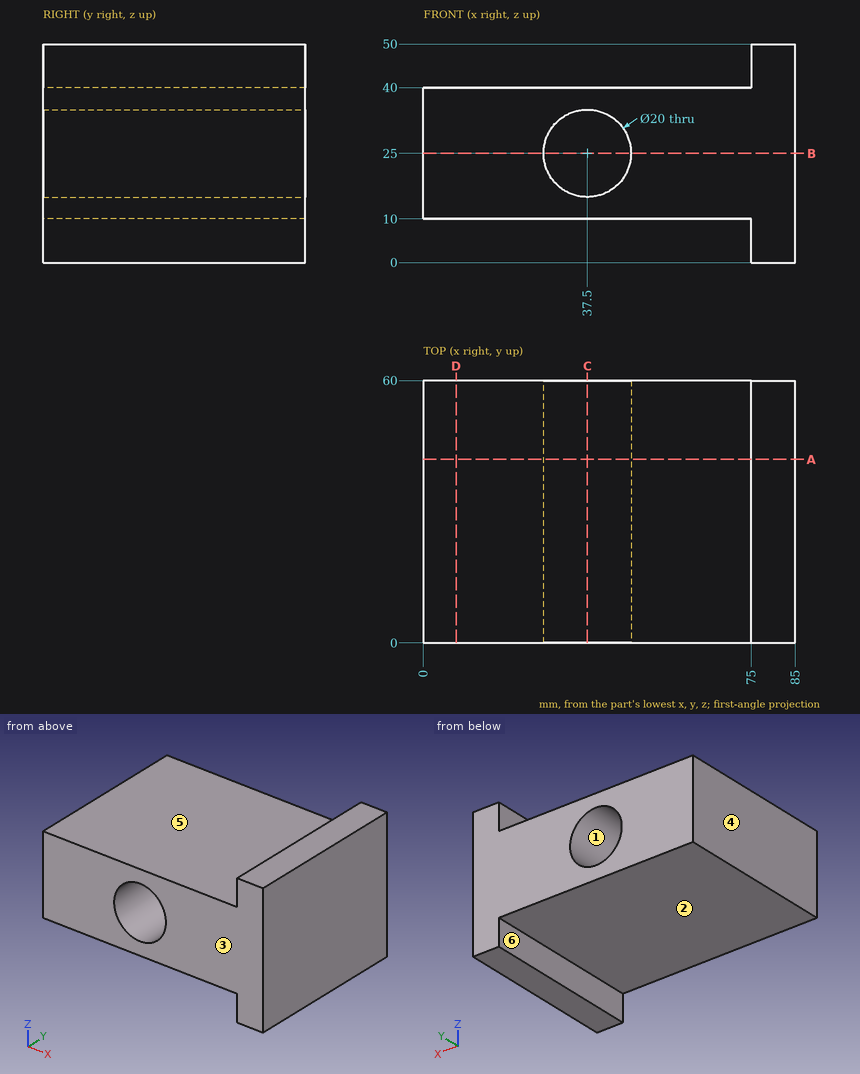
The figure shows three views and two pictorial views of one solid part (mm, origin at its lowest corner). Answer the questions. A direction names the side the tool comes from. Coordinates: 2 decimals unless noted, no trailing zeros. Loops run counter-clockwise (first coordinate to the right, second up) from the corner with the lowest first, then second, coordinate; pieces in that order, holes last. Notation, with made-up numbers: (69.5, 21.5) -> (107.5, 21.5) arc R22 ccw to (107.5, 29.5) -> close; hole circle Ø6 at (16.5, 5). An arc over 180 degrees is marked (long way). Write item = value, one per line. Start each with the question number.
1) A cutting plane is placed at D-D (x = 7.5). Give the vertices of the cut face in (y, z).
2) Straight lines are drawn through the part: line 1 (Z direction, x = 37.5, y = 44.5); line 2 (Z direction, x = 60, y = 21.5); line 3 (X direction, y = 45.5, z = 18). For each, find the intervals that lie inside material, in ascending order. Write a range as from..to.
3) The mould has two halves that part along Z. Classify the marked faces 1, 2 and 3: released by +Z, released by -Z, zero draft, split by the parting line, or undercut.
4) A cutting plane is placed at C-C (x = 37.5). Give the vertices of the cut face in (y, z), then the cut area to 3 significant figures.
5) Given pin 1 Ø6 at (x, y) = (45, 14) entering from -Z; pin 2 Ø8 at (x, y) = (18, 38.5) entering from +Z; pin 3 Ø8 at (y, z) = (25.5, 43.5) entering from -X; pin 4 Ø3 at (y, z) = (42.5, 6) entering from -X, each flat-ended and moving along its own axis, determine where each tip first touches the part or whether it passes through.
6) A cutting plane is placed at A-A (y = 42). Give the vertices of the cut face in (x, z), then the cut area to 3 significant figures.
7) A cutting plane is placed at B-B (z = 25). Give the vertices of the cut face in (x, y), then the cut area to 3 significant figures.
8) A tool of negligible diameter and unlimited length cuts with its end or side. For the marked faces 4, 5 and 6, from which of +Z, -Z, +X, -X, +Y, -Y can it reach the whole face along a straight path? Write none if from no direction.
Responses:
q1.outline = (0, 10) -> (60, 10) -> (60, 40) -> (0, 40) -> close
q2.line_1 = 10..15, 35..40
q2.line_2 = 10..40
q2.line_3 = 0..30.36, 44.64..85
q3.face_1 = undercut
q3.face_2 = released by -Z
q3.face_3 = zero draft
q4.outline = (0, 10) -> (60, 10) -> (60, 15) -> (0, 15) -> close; (0, 35) -> (60, 35) -> (60, 40) -> (0, 40) -> close
q4.area = 600 mm²
q5.pin_1 = 10
q5.pin_2 = 40
q5.pin_3 = 0
q5.pin_4 = 75
q6.outline = (0, 10) -> (75, 10) -> (75, 0) -> (85, 0) -> (85, 50) -> (75, 50) -> (75, 40) -> (0, 40) -> close; hole circle Ø20 at (37.5, 25)
q6.area = 2,440 mm²
q7.outline = (0, 0) -> (27.5, 0) -> (27.5, 60) -> (0, 60) -> close; (47.5, 0) -> (85, 0) -> (85, 60) -> (47.5, 60) -> close
q7.area = 3,900 mm²
q8.face_4 = +Z, -Z, -X, +Y, -Y
q8.face_5 = +Z, -X, +Y, -Y
q8.face_6 = -Z, -X, +Y, -Y
